```python
from build123d import *

# Parameters (mm, degrees)
F1_DEPTH = 32.004
F3_DEPTH = 76.54355
F4_R     = 1.778
F5_DEPTH = 44.60469
F7_DEPTH = 32.004


# Not quite as in the source:
# - ends of sketch curves that miss each other by under 0.0002 mm in the source are joined


with BuildPart() as f1:
    # F0 (on Top) → F1 (new body)
    with BuildSketch(Plane.XY):
        with BuildLine():
            Line((-6.8850605494, 65.9121533447), (-6.8850605494, 61.0852363653))
            ThreePointArc((-6.8850605494, 61.0852363653), (-22.2043438922, 46.3803648051), (-27.8400605494, 25.9071533447))
            ThreePointArc((-27.8400605494, 25.9071533447), (-23.8462320221, 8.4831597105), (-12.6621800762, -5.4618466553))
            Line((-12.6621800762, -5.4618466553), (-75.5756720901, -5.4618466553))
            Line((-75.5756720901, -5.4618466553), (-75.5756720901, -14.0978466553))
            Line((-75.5756720901, -14.0978466553), (12.1649394506, -14.0978466553))
            ThreePointArc((12.1649394506, -14.0978466553), (40.452746232, -2.3806534366), (52.1699394506, 25.9071533447))
            ThreePointArc((52.1699394506, 25.9071533447), (46.5342227935, 46.3803648051), (31.2149394506, 61.0852363653))
            Line((31.2149394506, 61.0852363653), (31.2149394506, 65.9121533447))
            Line((31.2149394506, 65.9121533447), (12.1649394506, 65.9121533447))
            Line((12.1649394506, 65.9121533447), (-6.8850605494, 65.9121533447))
        make_face()
        with BuildLine():
            Line((-5.8923298493, -10.2878466553), (-5.8923298493, -5.4618466553))
            ThreePointArc((-5.8923298493, -5.4618466553), (-19.1692254039, 7.7895338028), (-24.0300605494, 25.9071533447))
            ThreePointArc((-24.0300605494, 25.9071533447), (12.1649394506, 62.1021533447), (48.3599394506, 25.9071533447))
            ThreePointArc((48.3599394506, 25.9071533447), (37.7586693957, 0.3134233997), (12.1649394506, -10.2878466553))
            Line((12.1649394506, -10.2878466553), (-5.8923298493, -10.2878466553))
        make_face(mode=Mode.SUBTRACT)
    extrude(amount=F1_DEPTH)

    # F2 (on face) → F3 (cut)
    with BuildSketch(Plane(origin=(-75.5756720901, 0, 0), x_dir=(0, -1, 0), z_dir=(-1, 0, 0))):
        with BuildLine():
            Line((5.4618466553, 28.702), (5.4618466553, 3.302))
            ThreePointArc((5.4618466553, 3.302), (10.2879432961, 16.002), (5.4618466553, 28.702))
        make_face()
    extrude(amount=-F3_DEPTH, mode=Mode.SUBTRACT)

    # F4 (on face) → F5 (cut)
    with BuildSketch(Plane(origin=(0, 65.9121533447, 0), x_dir=(-1, 0, 0), z_dir=(0, 1, 0))):
        with Locations((-25.6732087171, 22.4042255431)):
            Circle(F4_R)
        with Locations((-25.6569720394, 28.7826433778)):
            Circle(F4_R)
        with Locations((-25.6396394506, 16.002)):
            Circle(F4_R)
        with Locations((-25.6375241614, 9.5933126286)):
            Circle(F4_R)
        with Locations((-25.6380084491, 3.1869229861)):
            Circle(F4_R)
        with Locations((1.3113915509, 3.1869229861)):
            Circle(F4_R)
        with Locations((1.3118758386, 9.5933126286)):
            Circle(F4_R)
        with Locations((1.3097605494, 16.002)):
            Circle(F4_R)
        with Locations((1.2761912829, 22.4042255431)):
            Circle(F4_R)
        with Locations((1.2924279606, 28.7826433778)):
            Circle(F4_R)
    extrude(amount=-F5_DEPTH, mode=Mode.SUBTRACT)

    # F6 (on face) → F7 (join)
    with BuildSketch(Plane.XY.offset(32.004)):
        with BuildLine():
            ThreePointArc((-24.5815716288, 41.7215122786), (-45.7821906846, 13.486402418), (-75.5756720901, -5.4618466553))
            Line((-75.5756720901, -5.4618466553), (-12.6621800762, -5.4618466553))
            ThreePointArc((-12.6621800762, -5.4618466553), (-23.9121515851, 16.7934110455), (-24.5815716288, 41.7215122786))
        make_face()
    extrude(amount=-F7_DEPTH)


solid = f1.part
```
Design review of the part built by this model. Coordinates are the model's own, in mm. A direction names the side the tool comes from. Round coordinates to 2 decimals unless told otherwise and drop trailing zeros. Write each loop counter-clockwise with the first axis right and the second up, starting at its lowest first coordinate (ties: lowest second). Pieces come first, ordered by that corner, then holes. Notation, with made-up numbers: (-35, 69.5) -> (3, 69.5) arc R13 cw to (3, 85.5) -> close; hole circle Ø9 at (-33, -38.5). An arc over 180 degrees is marked (long way). Write item = value, one per line. Start each with the question number.
1) Wall thickness on probe 1 along Z at (x, y) = (-1, 61.5); probe 2 along Y at (x, z) = (-9.5, 10.5); probe 3 along Y at (x, z) = (-26, 16.5): over which ranges is each line inside the solid? List them lowest first. Write a range as from..to.
2) Clearance check with flat-ended pins moving along their axes: pin 1 (1 mm diameter, centred on y = 15, z = 3, fed in from +X); pin 2 (4 mm diameter, centred on y = -8.5, z = 24.5, fed in from +X); pin 3 (3 mm diameter, centred on x = 25.64, z = 9.59, fed in from -Y); pin 4 (5.5 mm diameter, centred on x = -0.5, z = 23.5, fed in from +Y). State where each tip first meets the part, or that it passes through.
3) Mouldability with a two-part tool opening along X and no side actions: class faces 4 (the face through (31.215, 63, 16)), 5 (the face through (12, 65.912, 16)), 6 (the face through (-5.892, -8, 4)) as +X half, -X half, draft (parallel to the pull), parting line (faces both ways), or undercut.
4) Take a section at B-B, the plane y = -9. State the section outline as (x, z) points.
5) Take a section at C-C, the plane x = 15.5. State the section outline as (y, z) points.
6) Take a section at D-D, the plane y = 39.5. State the section outline as (x, z) points, plus the area to 3 significant figures.
7) Tool access review of faces 1 (the face through (-41, -5.462, 16)), 2 (the face through (-3.006, 62.372, 16.536)), 3 (the face through (3, -10.288, 16)): name each direction out of +Z, -Z, +X, -X, +Y, -Y from which nothing blocks a thin tool from reaching the whole face with its end or side.
8) Take a section at A-A, the plane x = -20. State the section outline as (y, z) points, plus the area to 3 significant figures.
Results list:
q1.probe_1 = 0..1.44, 4.94..7.84, 11.34..14.25, 17.75..20.65, 24.16..27.03, 30.54..32
q1.probe_2 = -14.1..-9.48, -5.46..-3.09, 54.9..59.54
q1.probe_3 = -14.1..-10.28, -5.46..38.99
q2.pin_1 = 50.79
q2.pin_2 = 35.62
q2.pin_3 = -12.26
q2.pin_4 = 65.91
q3.face_4 = +X half
q3.face_5 = draft
q3.face_6 = undercut
q4.outline = (-75.58, 0) -> (-5.89, 0) -> (-5.89, 9.1) -> (-75.58, 9.1) -> close; (-75.58, 22.9) -> (-5.89, 22.9) -> (-5.89, 32) -> (-75.58, 32) -> close; (21.73, 0) -> (31.71, 0) -> (31.71, 32) -> (21.73, 32) -> close
q5.outline = (-13.96, 0) -> (-10.13, 0) -> (-10.13, 32) -> (-13.96, 32) -> close; (61.95, 0) -> (65.91, 0) -> (65.91, 32) -> (61.95, 32) -> close
q6.outline = (-25.73, 0) -> (-21.38, 0) -> (-21.38, 32) -> (-25.73, 32) -> close; (45.71, 0) -> (49.79, 0) -> (49.79, 32) -> (45.71, 32) -> close
q6.area = 270 mm²
q7.face_1 = -X
q7.face_2 = +Y
q7.face_3 = +Z, -Z
q8.outline = (-14.1, 0) -> (9.31, 0) -> (9.31, 32) -> (-14.1, 32) -> close; (42.51, 0) -> (49.69, 0) -> (49.69, 32) -> (42.51, 32) -> close; hole (-5.46, 3.3) -> (-5.46, 28.7) arc R19.12 ccw to start
q8.area = 895 mm²
